```python
from build123d import *

# Parameters (mm, degrees)
F0_R     = 19.05
F1_DEPTH = 22.225
F2_R     = 19.05
F2_R_2   = 6.35
F3_DEPTH = 9.525
F4_SIZE  = 0.635


with BuildPart() as f1:
    # F0 (on Front) → F1 (new body)
    with BuildSketch(Plane.XZ):
        Circle(F0_R)
    extrude(amount=F1_DEPTH)

    # F2 (on face) → F3 (cut)
    with BuildSketch(Plane(origin=(0, 0, 0), x_dir=(-1, 0, 0), z_dir=(0, 1, 0))):
        Circle(F2_R)
        Circle(F2_R_2, mode=Mode.SUBTRACT)
    extrude(amount=-F3_DEPTH, mode=Mode.SUBTRACT)

    # F4
    f4_edges = [f1.edges().sort_by_distance(p)[0] for p in [
        (6.35, 0, 0),
        (-19.05, -22.225, 0),
    ]]
    chamfer(f4_edges, length=F4_SIZE)


solid = f1.part
```
Model file for the job. Use its own axes, mm. A direction names the side the tool comes from. Coordinates: 2 decimals unless noted, no trailing zeros. Loops run counter-clockwise (first coordinate to the right, second up) from the corner with the lowest first, then second, coordinate; pieces in that order, holes last. Notation, with made-up numbers: (9.25, 30.5) -> (53.25, 30.5) arc R15 cw to (53.25, 57.5) -> close; hole circle Ø8 at (87, 8). An arc over 180 degrees is marked (long way). Answer as a JSON object with one key per item and string values.
Q1. Cut at D-D (y = -8.25). List the corners of the cut face in (x, z), and give its area (3 significant figures).
Report:
{"outline": "circle Ø12.7 at (0, 0)", "area": "127 mm2"}
Q2. Probe probe 1 along Y at (x, z) = (0.5, 7) (3 decimals); probe 2 along Z at (x, y) = (8, -12.25); probe 3 along Z at (x, y) = (-12.5, -20.25). List the from-to ranges inside material, lowest first.
Report:
{"probe 1": "y = -22.225 to -9.525", "probe 2": "z = -17.29 to 17.29", "probe 3": "z = -14.38 to 14.38"}
Q3. Cut at C-C (y = -18). List the corners of the cut face in (x, z).
Report:
{"outline": "circle Ø38.1 at (0, 0)"}
Q4. Cut at A-A (z = 0). List the corners of the cut face in (x, y) (3 decimals), and give its area (3 significant figures).
Report:
{"outline": "(-19.05, -21.59) -> (-18.415, -22.225) -> (18.415, -22.225) -> (19.05, -21.59) -> (19.05, -9.525) -> (6.35, -9.525) -> (6.35, -0.635) -> (5.715, 0) -> (-5.715, 0) -> (-6.35, -0.635) -> (-6.35, -9.525) -> (-19.05, -9.525) -> close", "area": "604 mm2"}
Q5. 3-axis set-ups, long thin cutter, end or side, ignore diameter. For faces 1 (the flat face through (0, -22.225, 0)), 2 (the cylindrical face through (1.38, -5.02, -6.2)): which of +Z, -Z, +X, -X, +Y, -Y reach the whole face in a straight line?
Report:
{"face 1": "+Z, -Z, +X, -X, -Y", "face 2": "+Y"}
Q6. Cut at B-B (x = 0). List the corners of the cut face in (y, z) (3 decimals).
Report:
{"outline": "(-22.225, -18.415) -> (-21.59, -19.05) -> (-9.525, -19.05) -> (-9.525, -6.35) -> (-0.635, -6.35) -> (0, -5.715) -> (0, 5.715) -> (-0.635, 6.35) -> (-9.525, 6.35) -> (-9.525, 19.05) -> (-21.59, 19.05) -> (-22.225, 18.415) -> close"}
Q7. Flat gauge pins, fed straight in: P1, Ø6, axis at x = 4.5, y = -6, coming from the +Z side; P2, Ø6, axis at y = -9.5, z = 12.5, coming from the +X side; P3, Ø2, axis at x = -10, z = -1, coming from the +Y side (3 decimals). Where does each tip first touch, or does it go through?
Report:
{"P1": "stops at z = 6.17", "P2": "stops at x = 16.51", "P3": "stops at y = -9.525"}
